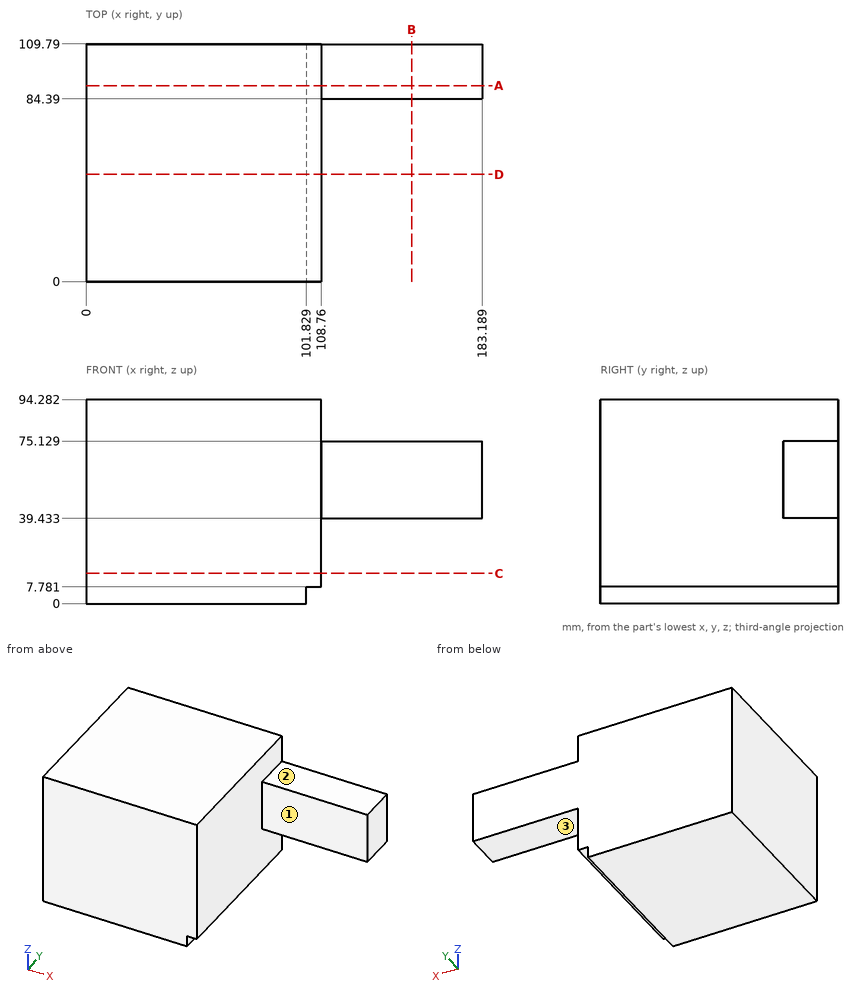
Geometry check sheet. Reference: drawing and pictorial views, mm from the part's lowest x, y, z. A direction names the side the tool comes from. Round coordinates to 2 decimals unless told otherwise and drop trailing zeros. Order: outer loops, then holes, each group sorted by start corner. A loop starts at its lowest first (then second) coordinate and runs counter-clockwise, first axis right, second up. Notation, with made-up numbers: M 70.5,68.5 L 80.5,68.5 A8 ccw 80.5,72.5 Z; hole C 64.25,15.5 d7. An arc over 180 degrees is marked long. One line per item, written item: value. Start each with the question number.
1. Section check A-A on y = 90.5. Enter the section's corners in (x, z).
2. Section check B-B on x = 150.5. Enter the section's corners in (y, z).
3. Section check D-D on y = 49.5. Enter the section's corners in (x, z), and give its area (3 significant figures).
4. Access from +Z, -Z, +X, -X, +Y, -Y to the whole of each face (thin tool, end or side, straight path). Record for the marked faces 1, 2 and 3.
5. Scan lines: line 1 along Z through (x, y) = (159.5, 105.5); line 2 along X through (y, z) = (28, 69.5); line 3 along X through (y, z) = (92.5, 7). Record each from-to range of solid material in increasing order.
6. Gauge pin test, flat ends, axial feed: P1, Ø20.5, axis at x = 141.5, y = 98.5, coming from the +Z side; P2, Ø8.5, axis at y = 45.5, z = 2, coming from the +X side; P3, Ø18, axis at x = 152, z = 61, coming from the -Y side. Record the tip position at first contact, or that the pin passes through.
7. Section check C-C on z = 14. Enter the section's corners in (x, y).
Results found:
1. outline: M 0,0 L 101.83,0 L 101.83,7.78 L 108.76,7.78 L 108.76,39.43 L 183.19,39.43 L 183.19,75.13 L 108.76,75.13 L 108.76,94.28 L 0,94.28 Z
2. outline: M 84.39,39.43 L 109.79,39.43 L 109.79,75.13 L 84.39,75.13 Z
3. outline: M 0,0 L 101.83,0 L 101.83,7.78 L 108.76,7.78 L 108.76,94.28 L 0,94.28 Z
3. area: 10,200 mm^2
4. face 1: +Z, -Z, +X, -Y
4. face 2: +Z, +X, +Y, -Y
4. face 3: -Z, +X, +Y, -Y
5. line 1: 39.43 to 75.13
5. line 2: 0 to 108.76
5. line 3: 0 to 101.83
6. P1: z = 75.13
6. P2: x = 101.83
6. P3: y = 84.39
7. outline: M 0,0 L 108.76,0 L 108.76,109.79 L 0,109.79 Z
